from build123d import *

# Parameters (mm, degrees)
SKETCH1_R           = 7
BOSS_EXTRUDE1_DEPTH = 4.5


with BuildPart() as part:
    # Sketch1 → Boss-Extrude1 (new, symmetric)
    with BuildSketch(Plane(origin=(0, 0, 0), x_dir=(1, 0, 0), z_dir=(0, 1, 0))):
        with BuildLine():
            Line((-1.254341559, 11.934262744), (-28.289662127, 9.092736051))
            ThreePointArc((-28.289662127, 9.092736051), (-43.850490966, 9.48747573), (-58.786122703, 13.871779345))
            ThreePointArc((-58.786122703, 13.871779345), (-74.520010862, 15.355444557), (-88, 7.106420865))
            Line((-88, 7.106420865), (-86.5, 4.508344654))
            Line((-86.5, 4.508344654), (-81.303847577, 7.508344654))
            Line((-81.303847577, 7.508344654), (-76.107695155, 4.508344654))
            Line((-76.107695155, 4.508344654), (-66.705771366, -11.776265037))
            ThreePointArc((-66.705771366, -11.776265037), (-56.482680545, -7.851988144), (-45.547275152, -7.278887832))
            Line((-45.547275152, -7.278887832), (-1.254341559, -11.934262744))
            ThreePointArc((-1.254341559, -11.934262744), (12, 0), (-1.254341559, 11.934262744))
        make_face()
        with Locations(Location((0, 0, 0), (0, 0, 270))):
            Circle(SKETCH1_R, mode=Mode.SUBTRACT)
        Polygon((-69.509618943, 5.080141424), (-63.509618943, -5.312163422), (-56.581415713, -1.312163422), (-62.581415713, 9.080141424), align=None, mode=Mode.SUBTRACT)
    extrude(amount=BOSS_EXTRUDE1_DEPTH, both=True)


solid = part.part
Model file for the job. Use its own axes, mm. A direction names the side the tool comes from. Round coordinates to 2 decimals unless told otherwise and drop trailing zeros. Loops run counter-clockwise (first coordinate to the right, second up) from the corner with the lowest first, then second, coordinate; pieces in that order, holes last. Notation, with made-up numbers: (2, 53.5) -> (10, 53.5) arc R16 cw to (10, 71.5) -> close; hole circle Ø5 at (78.5, 20.25). An arc over 180 degrees is marked (long way). Answer as CSV lines item,"result". Start each with the question number.
1) Probe line 1 along Z through (x, y) = (-69, 0.5); line 2 along X through (y, z) = (-0.75, 6.25); line 3 along X through (y, z) = (3.25, -0.75). List the from-to ranges inside material, lowest first.
2) Slice it at B-B (z = 2.75). List the corners of the cut face in (x, y), plus the area to 3 significant figures.
3) Slice it at A-A (x = 0). List the corners of the cut face in (y, z), plus the area to 3 significant figures.
4) Slice it at C-C (y = 2). List the corners of the cut face in (x, z).
5) Pin check, flat tips, straight feed: P1, Ø3, axis at y = -2, z = -11, coming from the +X side; P2, Ø4, axis at y = 1, z = -10, coming from the +X side; P3, Ø1.5, axis at y = 0.5, z = 3, coming from the +X side; P4, Ø12.5, axis at x = 0, z = 0, coming from the +Y side. Stop position of each tip, or through.
6) Tool access for faces 1 (the face through (-83.938, 0.063, -5.987)), 2 (the face through (-60.09, 0.06, 3.34)), 3 (the face through (-14.583, 0.063, -10.533)), 4 (the face through (-71.473, 0.063, 3.52)), 5 (the face through (-39, 4.5, -2)): list every direction of +Z, -Z, +X, -X, +Y, -Y with a clear straight run to the whole face (end or side of a thin tool).
7) Slice it at D-D (z = -2.25). List the corners of the cut face in (x, y), plus the area to 3 significant figures.
8) Mould opens along Z. For faces 6 (the face through (-39, -4.5, -2)), 7 (the face through (12, 0, 0)), 8 (the face through (-59.54, 0.06, -3.81)) say: +Z half, -Z half, draft (parallel to the pull), parting line (faces both ways), or undercut.
Filled in:
1,line 1,"z = -16 to -5.37, -4.2 to 7.8"
1,line 2,"x = -69.9 to -3.15, 3.15 to 10.24"
1,line 3,"x = -73.94 to -67.01, -57.77 to -6.96, 6.96 to 11.98"
2,outline,"(-71.92, -4.5) -> (-64.99, -4.5) -> (-64.99, 4.5) -> (-71.92, 4.5) -> close; (-59.07, -4.5) -> (-6.44, -4.5) -> (-6.44, 4.5) -> (-59.07, 4.5) -> close; (6.44, -4.5) -> (11.68, -4.5) -> (11.68, 4.5) -> (6.44, 4.5) -> close"
2,area,"583 mm2"
3,outline,"(-4.5, -12) -> (4.5, -12) -> (4.5, -7) -> (-4.5, -7) -> close; (-4.5, 7) -> (4.5, 7) -> (4.5, 12) -> (-4.5, 12) -> close"
3,area,"90.0 mm2"
4,outline,"(-88, -7.11) arc R25 ccw to (-58.79, -13.87) arc R60 cw to (-28.29, -9.09) -> (-1.25, -11.93) arc R12 ccw (long way) to (-1.25, 11.93) -> (-45.55, 7.28) arc R35 cw to (-66.71, 11.78) -> (-76.11, -4.51) -> (-81.3, -7.51) -> (-86.5, -4.51) -> close; hole (-69.51, -5.08) -> (-62.58, -9.08) -> (-56.58, 1.31) -> (-63.51, 5.31) -> close; hole circle Ø14 at (0, 0)"
5,P1,"stops at x = 7.33"
5,P2,"stops at x = 8.94"
5,P3,"stops at x = 11.79"
5,P4,"passes through"
6,face 1,"+Z, +Y, -Y"
6,face 2,"+Y, -Y"
6,face 3,"-Z, +Y, -Y"
6,face 4,"+Z, -X, +Y, -Y"
6,face 5,"+Z, -Z, +X, -X, +Y"
7,outline,"(-74.8, -4.5) -> (-67.88, -4.5) -> (-67.88, 4.5) -> (-74.8, 4.5) -> close; (-58.64, -4.5) -> (-6.63, -4.5) -> (-6.63, 4.5) -> (-58.64, 4.5) -> close; (6.63, -4.5) -> (11.79, -4.5) -> (11.79, 4.5) -> (6.63, 4.5) -> close"
7,area,"577 mm2"
8,face 6,"draft"
8,face 7,"parting line"
8,face 8,"undercut"
